CAD build for the part. Positions are in the model's coordinates, mm. Round coordinates to 2 decimals unless told otherwise and drop trailing zeros. Loops run counter-clockwise (first coordinate to the right, second up) from the corner with the lowest first, then second, coordinate; pieces in that order, holes last.
```python
from build123d import *

# Parameters (mm, degrees)
SKETCH1_R           = 1.5
SKETCH1_R_2         = 1
BOSS_EXTRUDE1_DEPTH = 0.8


with BuildPart() as part:
    # Sketch1 → Boss-Extrude1 (new body)
    with BuildSketch(Plane.XY):
        with BuildLine():
            Line((271.490097916, 97.17699679), (276.199648247, 80.675234569))
            ThreePointArc((276.199648247, 80.675234569), (280.131732963, 77.621186661), (284.059750771, 80.680463526))
            Line((284.059750771, 80.680463526), (288.244841789, 97.204357374))
            ThreePointArc((288.244841789, 97.204357374), (288.290696471, 97.447979301), (288.306060045, 97.695402532))
            Line((288.306060045, 97.695402532), (288.306060045, 105.52876871))
            ThreePointArc((288.306060045, 105.52876871), (286.84159395, 109.064302616), (283.306060045, 110.52876871))
            Line((283.306060045, 110.52876871), (273.41330701, 110.52876871))
            ThreePointArc((273.41330701, 110.52876871), (271.999093448, 109.942982273), (271.41330701, 108.52876871))
            Line((271.41330701, 108.52876871), (271.41330701, 97.725874534))
            ThreePointArc((271.41330701, 97.725874534), (271.43259777, 97.448762814), (271.490097916, 97.17699679))
        make_face()
        with Locations((280.129035475, 81.676015872)):
            Circle(SKETCH1_R, mode=Mode.SUBTRACT)
        with Locations((277.387391499, 105.581442102)):
            Circle(SKETCH1_R_2, mode=Mode.SUBTRACT)
        with Locations((277.387391499, 97.638982501)):
            Circle(SKETCH1_R_2, mode=Mode.SUBTRACT)
    extrude(amount=BOSS_EXTRUDE1_DEPTH)


solid = part.part
```
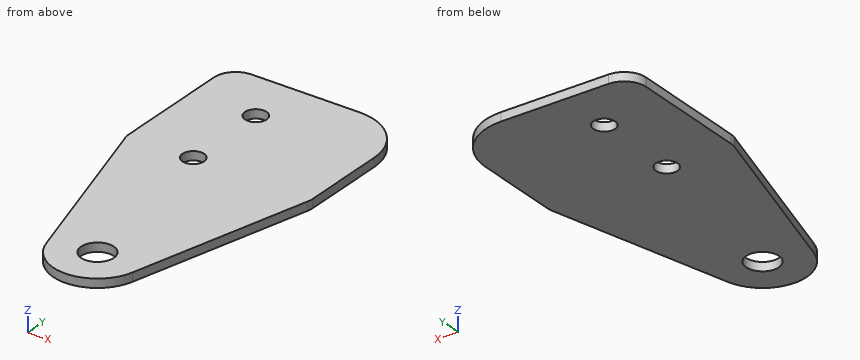
Item 1: Cut at D-D, the plane y = 87.5. Give the cut face in (x, z), plus the area to 3 significant figures.
Answers follow:
outline: (274.25, 0) - (285.79, 0) - (285.79, 0.8) - (274.25, 0.8) - close
area: 9.23 mm2
Item 2: Cut at B-B, the plane z = 0.15. Give the cut face in (x, y).
Answers follow:
outline: (271.41, 97.73) arc R2 ccw to (271.49, 97.18) - (276.2, 80.68) arc R4.05 ccw to (284.06, 80.68) - (288.24, 97.2) arc R2 ccw to (288.31, 97.7) - (288.31, 105.53) arc R5 ccw to (283.31, 110.53) - (273.41, 110.53) arc R2 ccw to (271.41, 108.53) - close; hole circle Ø2 at (277.39, 97.64); hole circle Ø2 at (277.39, 105.58); hole circle Ø3 at (280.13, 81.68)
Item 3: Cut at C-C, the plane y = 106. Give the cut face in (x, z), plus the area to 3 significant figures.
Answers follow:
outline: (271.41, 0) - (276.48, 0) - (276.48, 0.8) - (271.41, 0.8) - close; (278.3, 0) - (288.28, 0) - (288.28, 0.8) - (278.3, 0.8) - close
area: 12.0 mm2
Item 4: Cut at A-A, the plane x = 280.25. Give the cut face in (y, z), plus the area to 3 significant figures.
Answers follow:
outline: (77.62, 0) - (80.18, 0) - (80.18, 0.8) - (77.62, 0.8) - close; (83.17, 0) - (110.53, 0) - (110.53, 0.8) - (83.17, 0.8) - close
area: 23.9 mm2
Item 5: Probe line 1 (Y direction, x = 276.5, z = 0.5); line 2 (Y direction, x = 277.75, z = 0.7); line 3 (Y direction, x = 279.5, z = 0.5). List the from-to ranges inside material, lowest first.
Answers follow:
line 1: y = 79.87 to 97.18, 98.1 to 105.12, 106.04 to 110.53
line 2: y = 78.39 to 96.71, 98.57 to 104.65, 106.51 to 110.53
line 3: y = 77.67 to 80.31, 83.04 to 110.53
